```python
from build123d import *

# Parameters (mm, degrees)
SKETCH3_W                      = 50
SKETCH3_H                      = 100
BASE_FLANGE1_DEPTH             = 1
EDGE_FLANGE1_STRIP_W           = 6.2
EDGE_FLANGE1_STRIP_H           = 1
EDGE_FLANGE1_STRIP_CUT_DEPTH   = 50
EDGE_FLANGE1_STRIP_2_W         = 6.2
EDGE_FLANGE1_STRIP_2_H         = 1
EDGE_FLANGE1_STRIP_CUT_2_DEPTH = 50
EDGE_FLANGE1_DEPTH             = 50
EDGE_FLANGE1_BEND_DEPTH        = 50
EDGE_FLANGE2_STRIP_W           = 6.2
EDGE_FLANGE2_STRIP_H           = 1
EDGE_FLANGE2_STRIP_CUT_DEPTH   = 50
EDGE_FLANGE2_STRIP_2_W         = 6.2
EDGE_FLANGE2_STRIP_2_H         = 1
EDGE_FLANGE2_STRIP_CUT_2_DEPTH = 50
EDGE_FLANGE2_DEPTH             = 50
EDGE_FLANGE2_BEND_DEPTH        = 50
SKETCH20_R                     = 3
CUT_EXTRUDE1_DEPTH             = 94


# Sheet-metal steps are written as plain solids
with BuildPart() as part:
    # Sketch3 → Base-Flange1 (new body)
    with BuildSketch(Plane.XY):
        Rectangle(SKETCH3_W, SKETCH3_H)
    extrude(amount=-BASE_FLANGE1_DEPTH)

    # Edge-Flange1 strip (across the edge) → Edge-Flange1 strip cut (cut)
    with BuildSketch(Plane(origin=(-25, -50, 0), x_dir=(0, 1, 0), z_dir=(1, 0, 0))):
        with Locations((-1, -0.5)):
            Rectangle(EDGE_FLANGE1_STRIP_W, EDGE_FLANGE1_STRIP_H)
    extrude(amount=EDGE_FLANGE1_STRIP_CUT_DEPTH, mode=Mode.SUBTRACT)

    # Edge-Flange1 strip 2 (across the edge) → Edge-Flange1 strip cut 2 (cut)
    with BuildSketch(Plane(origin=(25, 50, 0), x_dir=(0, -1, 0), z_dir=(-1, 0, 0))):
        with Locations((-1, -0.5)):
            Rectangle(EDGE_FLANGE1_STRIP_2_W, EDGE_FLANGE1_STRIP_2_H)
    extrude(amount=EDGE_FLANGE1_STRIP_CUT_2_DEPTH, mode=Mode.SUBTRACT)

    # Edge-Flange1 section (across the edge) → Edge-Flange1 (add)
    with BuildSketch(Plane(origin=(-25, -50, 0), x_dir=(0, 1, 0), z_dir=(1, 0, 0))):
        with BuildLine():
            Line((0, 1.1), (0, 39))
            Line((0, 39), (1, 39))
            Line((1, 39), (1, 1.1))
            ThreePointArc((1, 1.1), (1.322182541, 0.322182541), (2.1, 0))
            Line((2.1, 0), (2.1, -1))
            ThreePointArc((2.1, -1), (0.61507576, -0.38492424), (0, 1.1))
        make_face()
    extrude(amount=EDGE_FLANGE1_DEPTH)

    # Edge-Flange1 section 2 (across the edge) → Edge-Flange1 bend (add)
    with BuildSketch(Plane(origin=(25, 50, 0), x_dir=(0, -1, 0), z_dir=(-1, 0, 0))):
        with BuildLine():
            Line((0, 1.1), (0, 39))
            Line((0, 39), (1, 39))
            Line((1, 39), (1, 1.1))
            ThreePointArc((1, 1.1), (1.322182541, 0.322182541), (2.1, 0))
            Line((2.1, 0), (2.1, -1))
            ThreePointArc((2.1, -1), (0.61507576, -0.38492424), (0, 1.1))
        make_face()
    extrude(amount=EDGE_FLANGE1_BEND_DEPTH)

    # Edge-Flange2 strip (across the edge) → Edge-Flange2 strip cut (cut)
    with BuildSketch(Plane(origin=(25, -50, 39), x_dir=(0, 0, -1), z_dir=(-1, 0, 0))):
        with Locations((-1, -0.5)):
            Rectangle(EDGE_FLANGE2_STRIP_W, EDGE_FLANGE2_STRIP_H)
    extrude(amount=EDGE_FLANGE2_STRIP_CUT_DEPTH, mode=Mode.SUBTRACT)

    # Edge-Flange2 strip 2 (across the edge) → Edge-Flange2 strip cut 2 (cut)
    with BuildSketch(Plane(origin=(-25, 50, 39), x_dir=(0, 0, -1), z_dir=(1, 0, 0))):
        with Locations((-1, -0.5)):
            Rectangle(EDGE_FLANGE2_STRIP_2_W, EDGE_FLANGE2_STRIP_2_H)
    extrude(amount=EDGE_FLANGE2_STRIP_CUT_2_DEPTH, mode=Mode.SUBTRACT)

    # Edge-Flange2 section (across the edge) → Edge-Flange2 (add)
    with BuildSketch(Plane(origin=(25, -50, 39), x_dir=(0, 0, -1), z_dir=(-1, 0, 0))):
        with BuildLine():
            Line((0, 1.1), (0, 14))
            Line((0, 14), (1, 14))
            Line((1, 14), (1, 1.1))
            ThreePointArc((1, 1.1), (1.322182541, 0.322182541), (2.1, 0))
            Line((2.1, 0), (2.1, -1))
            ThreePointArc((2.1, -1), (0.61507576, -0.38492424), (0, 1.1))
        make_face()
    extrude(amount=EDGE_FLANGE2_DEPTH)

    # Edge-Flange2 section 2 (across the edge) → Edge-Flange2 bend (add)
    with BuildSketch(Plane(origin=(-25, 50, 39), x_dir=(0, 0, -1), z_dir=(1, 0, 0))):
        with BuildLine():
            Line((0, 1.1), (0, 14))
            Line((0, 14), (1, 14))
            Line((1, 14), (1, 1.1))
            ThreePointArc((1, 1.1), (1.322182541, 0.322182541), (2.1, 0))
            Line((2.1, 0), (2.1, -1))
            ThreePointArc((2.1, -1), (0.61507576, -0.38492424), (0, 1.1))
        make_face()
    extrude(amount=EDGE_FLANGE2_BEND_DEPTH)

    # Sketch20 → Cut-Extrude1 (cut)
    with BuildSketch(Plane(origin=(0, 0, -1), x_dir=(-1, 0, 0), z_dir=(0, 0, -1))):
        with Locations((15, 42.9)):
            Circle(SKETCH20_R)
        with Locations((-15, 42.9)):
            Circle(SKETCH20_R)
        with Locations((15, 59)):
            Circle(SKETCH20_R)
        with Locations((-15, 59)):
            Circle(SKETCH20_R)
        with Locations((-15, -59)):
            Circle(SKETCH20_R)
        with Locations((15, -59)):
            Circle(SKETCH20_R)
        with Locations((15, -42.9)):
            Circle(SKETCH20_R)
        with Locations((-15, -42.9)):
            Circle(SKETCH20_R)
        with BuildLine():
            Line((8, 17.746865737), (8, -12.253134263))
            ThreePointArc((8, -12.253134263), (0, -20.253134263), (-8, -12.253134263))
            Line((-8, -12.253134263), (-8, 17.746865737))
            ThreePointArc((-8, 17.746865737), (0, 25.746865737), (8, 17.746865737))
        make_face()
    extrude(amount=-CUT_EXTRUDE1_DEPTH, mode=Mode.SUBTRACT)


solid = part.part
```
Geometry: final body of the model. Coordinates: model frame, mm. A direction names the side the tool comes from. Round coordinates to 2 decimals unless told otherwise and drop trailing zeros. Write each loop counter-clockwise with the first axis right and the second up, starting at its lowest first coordinate (ties: lowest second). Pieces come first, ordered by that corner, then holes. Notation, with made-up numbers: (39, 28) -> (80, 28) arc R7 cw to (80, 34) -> close; hole circle Ø11 at (-5.75, 15.5). An arc over 180 degrees is marked (long way). Return JSON: item names as keys, results as strings.
Q1. Section D-D on y = 42.9. Return the cut outline in (x, z), and give its area (3 significant figures).
From the geometry:
{"outline": "(-25, -1) -> (-18, -1) -> (-18, 0) -> (-25, 0) -> close; (-12, -1) -> (12, -1) -> (12, 0) -> (-12, 0) -> close; (18, -1) -> (25, -1) -> (25, 0) -> (18, 0) -> close", "area": "38.0 mm2"}
Q2. Mould query, pull axis Y, two halves, no side actions, for faces 1 (the flat face through (0, 50, 19)), 2 (the flat face through (0, 58, 38)), 3 (the cylindrical face through (15.391, 45.874, -0.507)). Classes: +Y half, -Y half, draft (parallel to the pull), parting line (faces both ways), or undercut.
From the geometry:
{"face 1": "+Y half", "face 2": "draft", "face 3": "undercut"}
Q3. Ray query, line 1 (Y direction, x = -15, z = -0.7); line 2 (Y direction, x = 7, z = 16); line 3 (Y direction, x = -15, z = 38.4). Return the intervals inside material, ascending.
From the geometry:
{"line 1": "-48.98 to -45.9, -39.9 to 39.9, 45.9 to 48.98", "line 2": "-50 to -49, 49 to 50", "line 3": "-64 to -62, -56 to -49.63, 49.63 to 56, 62 to 64"}
Q4. Set-up query: faces 4 (the flat face through (0, -58, 38)), 5 (the cylindrical face through (0.176, 25.745, -0.507)), 6 (the flat face through (25, 0.3, -0.4)), 7 (the flat face through (-11, 1, 0)), 8 (the flat face through (-25, 0.3, -0.4)). Return all of +Z, -Z, +X, -X, +Y, -Y with unobstructed straight access to the full face (end or side cutting, diameter ignored); none if empty.
From the geometry:
{"face 4": "-Z, +X, -X, -Y", "face 5": "+Z, -Z", "face 6": "+Z, -Z, +X, +Y, -Y", "face 7": "+Z, +X, -X", "face 8": "+Z, -Z, -X, +Y, -Y"}
Q5. First-contact query: pin 1 Ø1.5 at (x, z) = (-15.5, 31.5) entering from -Y; pin 2 Ø10.5 at (x, z) = (6.5, 24) entering from +Y; pin 3 Ø2 at (x, y) = (13, 33) entering from +Z; pin 4 Ø5 at (x, y) = (-15, 42.9) entering from -Z. Flat tips, straight axial feed; report the tip coordinate or a pass-through.
From the geometry:
{"pin 1": "y = -50", "pin 2": "y = 50", "pin 3": "z = 0", "pin 4": "through"}
Q6. Section C-C on x = 0. Return the cut outline in (y, z).
From the geometry:
{"outline": "(-64, 38) -> (-51.1, 38) arc R1.1 cw to (-50, 36.9) -> (-50, 1.1) arc R2.1 ccw to (-47.9, -1) -> (-20.25, -1) -> (-20.25, 0) -> (-47.9, 0) arc R1.1 cw to (-49, 1.1) -> (-49, 36.9) arc R2.1 ccw to (-51.1, 39) -> (-64, 39) -> close; (25.75, -1) -> (47.9, -1) arc R2.1 ccw to (50, 1.1) -> (50, 36.9) arc R1.1 cw to (51.1, 38) -> (64, 38) -> (64, 39) -> (51.1, 39) arc R2.1 ccw to (49, 36.9) -> (49, 1.1) arc R1.1 cw to (47.9, 0) -> (25.75, 0) -> close"}
Q7. Section B-B on y = -5. Return the cut outline in (x, z), and give its area (3 significant figures).
From the geometry:
{"outline": "(-25, -1) -> (-8, -1) -> (-8, 0) -> (-25, 0) -> close; (8, -1) -> (25, -1) -> (25, 0) -> (8, 0) -> close", "area": "34.0 mm2"}
Q8. Section A-A on z = 26. Return the cut outline in (x, y), and give its area (3 significant figures).
From the geometry:
{"outline": "(-25, -50) -> (25, -50) -> (25, -49) -> (-25, -49) -> close; (-25, 49) -> (25, 49) -> (25, 50) -> (-25, 50) -> close", "area": "100 mm2"}
